from build123d import *

# Parameters (mm, degrees)
F0_R          = 25.4
F1_DEPTH      = 406.4
F1_DEPTH_BACK = 25.4
F2_R          = 19.05
F3_DEPTH      = 355.6
F4_R          = 12.7
F5_DEPTH      = 25.401


with BuildPart() as f1:
    # F0 (on Top) → F1 (new body, two sides)
    with BuildSketch(Plane.XY) as f1_sk:
        Circle(F0_R)
    extrude(amount=-F1_DEPTH)
    extrude(f1_sk.sketch, amount=F1_DEPTH_BACK)

    # F2 (on Top) → F3 (cut)
    with BuildSketch(Plane.XY):
        Circle(F2_R)
    extrude(amount=-F3_DEPTH, mode=Mode.SUBTRACT)

    # F4 (on Top) → F5 (cut, through all)
    with BuildSketch(Plane.XY):
        Circle(F4_R)
    extrude(amount=F5_DEPTH, mode=Mode.SUBTRACT)


solid = f1.part
CAD build for the part. Positions are in the model's coordinates, mm. A direction names the side the tool comes from. Coordinates: 2 decimals unless noted, no trailing zeros. Order: outer loops, then holes, each group sorted by start corner. A loop starts at its lowest first (then second) coordinate and runs counter-clockwise, first axis right, second up.
Item 1: Drill centre lines: L1, parallel to Z at x = 7, y = 12; L2, parallel to Y at x = 0, z = 11.5; L3, parallel to X at y = 0.5, z = -275.5. Where is each one in solid material? Low to high.
Check sheet entries:
L1: z = -406.4 to -355.6, 0 to 25.4
L2: y = -25.4 to -12.7, 12.7 to 25.4
L3: x = -25.4 to -19.04, 19.04 to 25.4
Item 2: Band-saw the part on A-A on y = 0. List the corners of the cut face in (x, z), plus the area to 3 significant figures.
Check sheet entries:
outline: (-25.4, -406.4) - (25.4, -406.4) - (25.4, 25.4) - (12.7, 25.4) - (12.7, 0) - (19.05, 0) - (19.05, -355.6) - (-19.05, -355.6) - (-19.05, 0) - (-12.7, 0) - (-12.7, 25.4) - (-25.4, 25.4) - close
area: 7,740 mm2
Item 3: Two-plate mould, pull along X, no slides. Class faces 4 (the face through (5, 12, 25.4)), 5 (the face through (0, 0, -355.6)): +X half, -X half, draft (parallel to the pull), parting line (faces both ways), or undercut.
Check sheet entries:
face 4: draft
face 5: undercut
Item 4: Band-saw the part on C-C on z = -134. List the corners of the cut face in (x, y).
Check sheet entries:
outline: circle Ø50.8 at (0, 0); hole circle Ø38.1 at (0, 0)
Item 5: 3-axis set-ups, long thin cutter, end or side, ignore diameter. For faces 1 (the face through (0, 0, -406.4)), 2 (the face through (-2.75, -12.4, 12.52)), 3 (the face through (-15.12, -11.59, -175.31)): which of +Z, -Z, +X, -X, +Y, -Y reach the whole face in a straight line?
Check sheet entries:
face 1: -Z, +X, -X, +Y, -Y
face 2: +Z
face 3: none
Item 6: Pin check, flat tips, straight feed: pin 1 Ø1.5 at (x, z) = (1, -39.5) entering from -Y; pin 2 Ø2 at (x, z) = (-17.5, -111) entering from -Y; pin 3 Ø6 at (x, z) = (-19, -102.5) entering from -Y. Stop position of each tip, or through.
Check sheet entries:
pin 1: stops at y = -25.4
pin 2: stops at y = -19.31
pin 3: stops at y = -19.73
